Part model, mm, in its own coordinate system. A direction names the side the tool comes from. Round coordinates to 2 decimals unless told otherwise and drop trailing zeros. Loops run counter-clockwise (first coordinate to the right, second up) from the corner with the lowest first, then second, coordinate; pieces in that order, holes last. Notation, with made-up numbers: M -22.75,43 L 9.25,43 A30 ccw 9.25,69 Z; hole C 67.25,-5.5 d3. An arc over 180 degrees is marked long. Put each result on its own line as item: value. Start each with the question number.
1) Slice it at D-D on y = 61.5. Give the cut face in (x, z) (3 decimals), then the cut area to 3 significant figures.
2) Slice it at B-B on x = 7.5. Give the cut face in (y, z), then the cut area to 3 significant figures.
3) Which spindle directions (+Z, -Z, +X, -X, +Y, -Y) get a long thin tool onto all of the face, cutting with end or side? Do faces 5 (the flat face through (-4.445, -52, 32)), 6 (the flat face through (0.305, -52, 32)), 7 (the flat face through (0, -38, 34.924)), 8 (the cylindrical face through (-0.767, -32.257, 35.925)). Say none if no direction does.
4) Slice it at C-C on z = 32. Give the cut face in (x, y) (3 decimals), then the cut area to 3 significant figures.
5) Probe line 1 along Z through (x, y) = (6.5, -41.5); line 2 along Z through (x, y) = (2.5, 4); line 3 along Y through (x, z) = (7, 38.25). List the from-to ranges inside material, lowest first.
6) Drop flat-ended pins along their axis: pin 1 Ø5.5 at (x, y) = (4.5, -41.5) entering from +Z; pin 2 Ø2 at (x, y) = (7, 69) entering from -Z; pin 3 Ø2.5 at (x, z) = (-1.5, 34) entering from +Y. Give the stop position or say it passes through.
7) Pull direction Y, two halves, no side cores. Call faces 1 (the flat face through (0, 38, 49.528)), 2 (the flat face through (0, 84.962, 51)), 3 (the flat face through (-0.133, -16.662, 46.202)), 4 (the flat face through (-2, -50.292, 32)): +Y half, -Y half, draft (parallel to the pull), parting line (faces both ways), or undercut.
8) Slice it at A-A on y = -38.1. Give the cut face in (x, z) (3 decimals), then the cut area to 3 significant figures.
```python
from build123d import *

# Parameters (mm, degrees)
CYLINDER003_R     = 5.8928
CYLINDER003_DEPTH = 2.032
SKETCH003_W       = 19.05
SKETCH003_H       = 30.48
PAD_DEPTH         = 3.048
PAD001_DEPTH      = 19.05
SKETCH005_W       = 4.7498
SKETCH005_H       = 3.048
PAD002_DEPTH      = 9.398


with BuildPart() as part:
    # Cylinder003 → Cylinder003 (new body)
    with BuildSketch(Plane(origin=(0, -38.1, 34.923527), x_dir=(1, 0, 0), z_dir=(0, 0, 1))):
        Circle(CYLINDER003_R)
    extrude(amount=CYLINDER003_DEPTH)

    # Sketch003 → Pad (new body)
    with BuildSketch(Plane(origin=(0, -38.1, 36.955527), x_dir=(1, 0, 0), z_dir=(0, 0, 1))):
        Rectangle(SKETCH003_W, SKETCH003_H)
    extrude(amount=PAD_DEPTH)

    # Sketch004 → Pad001 (new body)
    with BuildSketch(Plane(origin=(-9.525, -38.1, 34.923527), x_dir=(0, -1, 0), z_dir=(-1, 0, 0))):
        Polygon((-15.24, 5.08), (-27.812359, 17.652359), (-123.062359, 17.652359), (-123.062359, 14.604359), (-27.812359, 14.604359), (-15.24, 2.032), align=None)
    extrude(amount=-PAD001_DEPTH)

    # Sketch005 → Pad002 (new body)
    with BuildSketch(Plane(origin=(0, -38.1, 36.955527), x_dir=(1, 0, 0), z_dir=(0, 0, -1))):
        with Locations((-2.0701, 13.716)):
            Rectangle(SKETCH005_W, SKETCH005_H)
    extrude(amount=PAD002_DEPTH)


solid = part.part
```
Recorded:
1. outline: M -9.525,49.528 L 9.525,49.528 L 9.525,52.576 L -9.525,52.576 Z
1. area: 58.1 mm2
2. outline: M -53.34,36.96 L -22.86,36.96 L -10.29,49.53 L 84.96,49.53 L 84.96,52.58 L -10.29,52.58 L -22.86,40 L -53.34,40 Z
2. area: 422 mm2
3. face 5: -Z, -X, -Y
3. face 6: -Z, +X, -Y
3. face 7: -Z, +X, -X, +Y
3. face 8: -Z
4. outline: M -4.445,-53.34 L 0.305,-53.34 L 0.305,-50.292 L -4.445,-50.292 Z
4. area: 14.5 mm2
5. line 1: z = 36.96 to 40
5. line 2: z = 49.53 to 52.58
5. line 3: y = -53.34 to -21.57
6. pin 1: stops at z = 40
6. pin 2: stops at z = 49.53
6. pin 3: stops at y = -32.24
7. face 1: draft
7. face 2: +Y half
7. face 3: -Y half
7. face 4: undercut
8. outline: M -9.525,36.956 L -5.893,36.956 L -5.893,34.924 L 5.893,34.924 L 5.893,36.956 L 9.525,36.956 L 9.525,40.004 L -9.525,40.004 Z
8. area: 82.0 mm2
